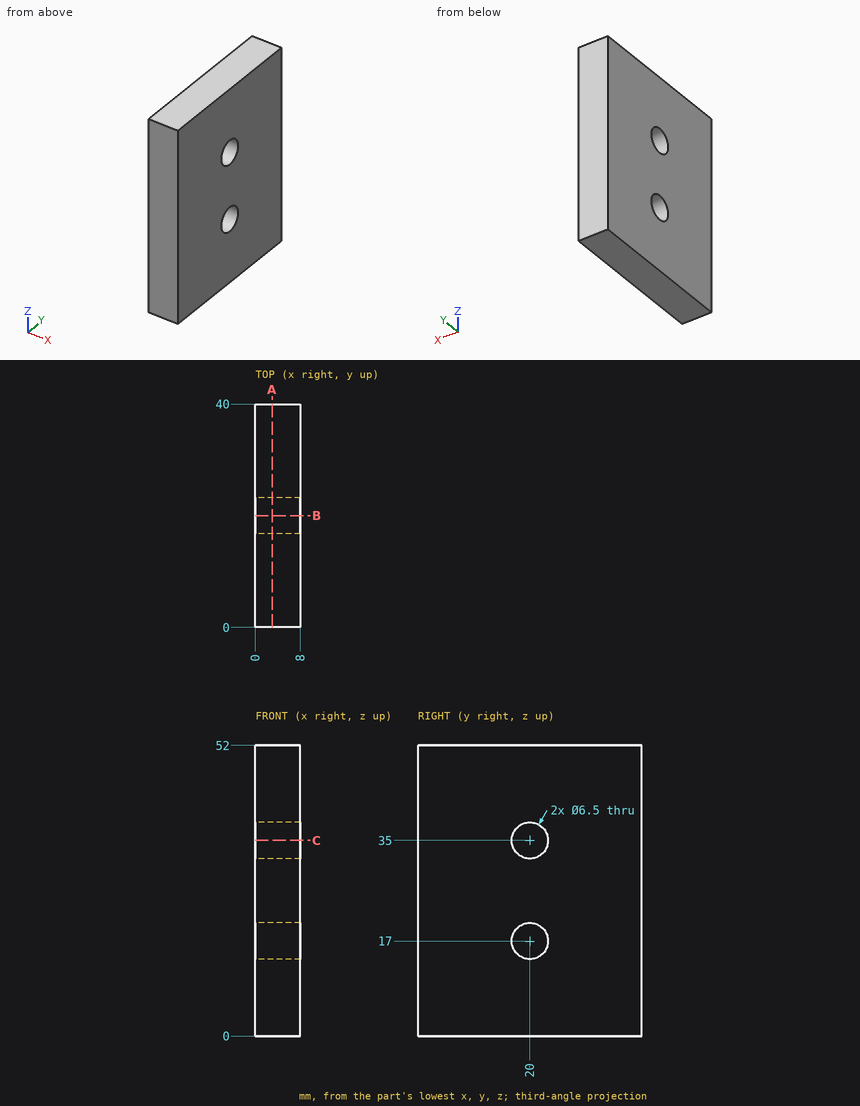
For this review, use the dimensioned drawing (mm, ordinates from the lowest corner) and the shaded views. Coordinates: 2 decimals unless noted, no trailing zeros. Order: outer loops, then holes, each group sorted by start corner. A loop starts at its lowest first (then second) coordinate and runs counter-clockwise, first axis right, second up. Notation, with made-up numbers: M 59.25,19 L 65.25,19 A14 ccw 65.25,25 Z; hole C -4,50.5 d4. An arc over 180 degrees is marked long. Answer as a JSON object with one key per item and string values. Group by question number.
1) Add section A-A, the plane x = 3. Write out the cut boundary in (y, z).
2) Add section C-C, the plane z = 35. Write out the cut boundary in (x, y).
3) Add section B-B, the plane y = 20. Write out the cut boundary in (x, z).
4) Wall thickness on L1, parallel to Y at x = 4.75, z = 17; L2, parallel to Z at x = 5.25, y = 20; L3, parallel to Z at x = 3.5, y = 23: over which ranges is each line inside the solid? List them lowest first.
Computed values:
{
 "1": {"outline": "M 0,0 L 40,0 L 40,52 L 0,52 Z; hole C 20,17 d6.5; hole C 20,35 d6.5"},
 "2": {"outline": "M 0,0 L 8,0 L 8,16.75 L 0,16.75 Z; M 0,23.25 L 8,23.25 L 8,40 L 0,40 Z"},
 "3": {"outline": "M 0,0 L 8,0 L 8,13.75 L 0,13.75 Z; M 0,20.25 L 8,20.25 L 8,31.75 L 0,31.75 Z; M 0,38.25 L 8,38.25 L 8,52 L 0,52 Z"},
 "4": {"L1": "y = 0 to 16.75, 23.25 to 40", "L2": "z = 0 to 13.75, 20.25 to 31.75, 38.25 to 52", "L3": "z = 0 to 15.75, 18.25 to 33.75, 36.25 to 52"}
}
